from build123d import *

# Parameters (mm, degrees)
F0_W     = 2200
F0_H     = 1500
F1_DEPTH = 300
F2_W     = 100
F2_H     = 100
F3_DEPTH = 300
F4_W     = 100
F4_H     = 1500
F5_DEPTH = 300
F6_R     = 100


with BuildPart() as f1:
    # F0 (on Top) → F1 (new body)
    with BuildSketch(Plane.XY):
        Rectangle(F0_W, F0_H)
    extrude(amount=F1_DEPTH)

    # F2 (on face) → F3 (join)
    with BuildSketch(Plane.XY.offset(300)):
        with Locations((-1050, -700)):
            Rectangle(F2_W, F2_H)
        with Locations((-1050, 700)):
            Rectangle(F2_W, F2_H)
        with Locations((1050, -700)):
            Rectangle(F2_W, F2_H)
        with Locations((1050, 700)):
            Rectangle(F2_W, F2_H)
    extrude(amount=F3_DEPTH)

    # F4 (on face) → F5 (join)
    with BuildSketch(Plane(origin=(0, 0, 0), x_dir=(1, 0, 0), z_dir=(0, 0, -1))):
        with Locations((1050, 0)):
            Rectangle(F4_W, F4_H)
    extrude(amount=F5_DEPTH)

    # F6
    f6_edges = [f1.edges().sort_by_distance(p)[0] for p in [
        (1050, -750, -300),
        (1050, 750, -300),
    ]]
    fillet(f6_edges, radius=F6_R)


solid = f1.part
Verification items for the finished model (mm, model axes). A direction names the side the tool comes from. Round coordinates to 2 decimals unless told otherwise and drop trailing zeros. Order: outer loops, then holes, each group sorted by start corner. A loop starts at its lowest first (then second) coordinate and runs counter-clockwise, first axis right, second up. Notation, with made-up numbers: (83, 88.5) -> (128, 88.5) arc R12 ccw to (128, 109.5) -> close; hole circle Ø5 at (-26.75, 67). An arc over 180 degrees is marked (long way). Put each result on its own line as item: value.
1) Section check A-A (z = 426). Record the cut outline in (x, y), then the cut area to 3 significant figures.
Final values:
outline: (-1100, -750) -> (-1000, -750) -> (-1000, -650) -> (-1100, -650) -> close; (-1100, 650) -> (-1000, 650) -> (-1000, 750) -> (-1100, 750) -> close; (1000, -750) -> (1100, -750) -> (1100, -650) -> (1000, -650) -> close; (1000, 650) -> (1100, 650) -> (1100, 750) -> (1000, 750) -> close
area: 40,000 mm^2
2) Section check C-C (x = 774). Record the cut outline in (y, z), then the cut area to 3 significant figures.
Final values:
outline: (-750, 0) -> (750, 0) -> (750, 300) -> (-750, 300) -> close
area: 450,000 mm^2
3) Mould release check, pull along Y, two halves, no side actions. Record for faces 1 (the flat face through (-1000, 699, 448)), 2 (the flat face through (1049, -650, 448)), 3 (the flat face through (-15, 750, 206)): +Y half, -Y half, draft (parallel to the pull), parting line (faces both ways), or undercut.
Final values:
face 1: draft
face 2: undercut
face 3: +Y half
4) Section check B-B (y = 34.5). Record the cut outline in (x, z).
Final values:
outline: (-1100, 0) -> (1000, 0) -> (1000, -300) -> (1100, -300) -> (1100, 300) -> (-1100, 300) -> close
5) Depth check by flat-ended pin: pin 1 (12 mm diameter, centred on x = 286, y = -59.5, fed in from -Z). Enter the tip coordinate at first touch or a pass-through.
Final values:
pin 1: stops at z = 0
6) Set-up check for faces 4 (the flat face through (-1051, -650, 448)), 5 (the flat face through (1000, 10, -148)), 6 (the flat face through (1000, -701, 448)): record each of +Z, -Z, +X, -X, +Y, -Y from which the full face is reachable in a straight line by a thin tool's end or side.
Final values:
face 4: +Z, +X, -X
face 5: -Z, -X, +Y, -Y
face 6: +Z, +Y, -Y
7) Material ranges on line 1 (X direction, y = -682, z = 450.5); line 2 (Z direction, x = -871, y = -428); line 3 (X direction, y = 510.5, z = -135), recorded low to high.
Final values:
line 1: x = -1100 to -1000, 1000 to 1100
line 2: z = 0 to 300
line 3: x = 1000 to 1100
